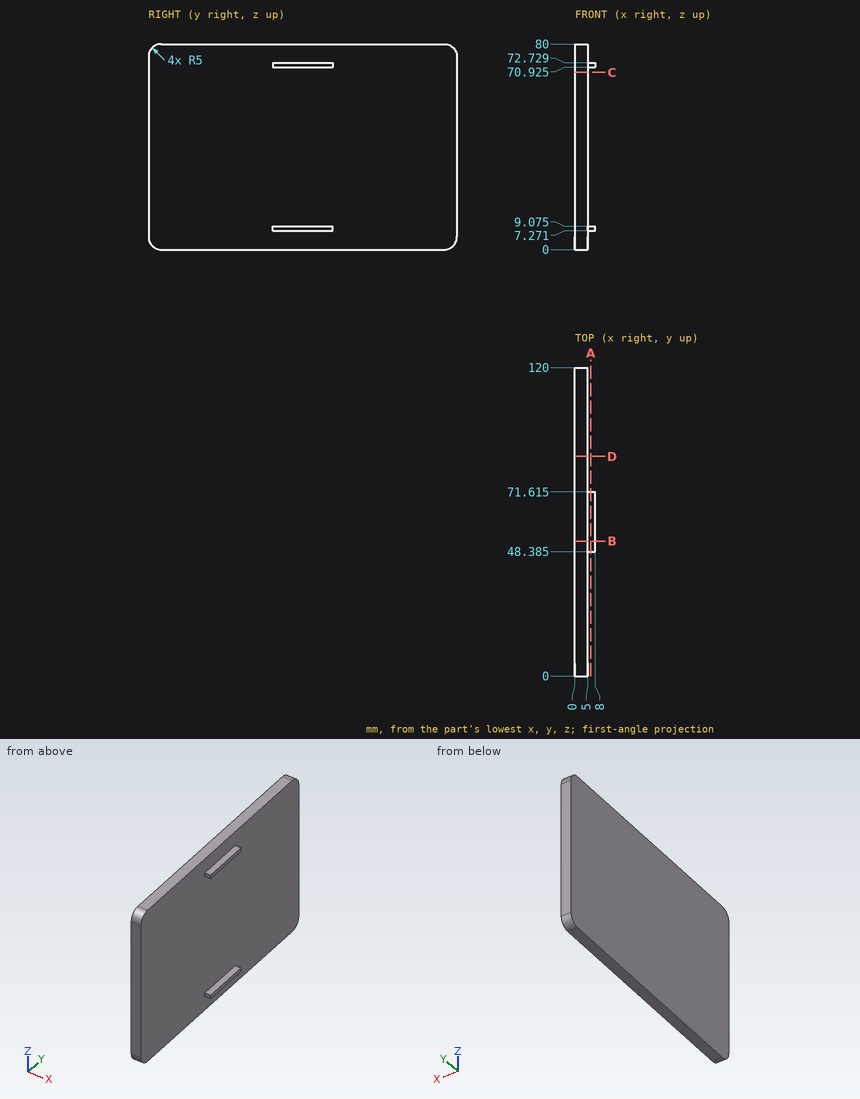
Job drawing, mm, ordinate dimensions from the low corner. One solid piece. Round coordinates to 2 decimals unless told otherwise and drop trailing zeros. Loops run counter-clockwise (first coordinate to the right, second up) from the corner with the lowest first, then second, coordinate; pieces in that order, holes last. Notation, with made-up numbers: (15.25, 2.5) -> (34.25, 2.5) arc R27 ccw to (34.25, 27.5) -> close; hole circle Ø2 at (73.25, 6). An arc over 180 degrees is marked (long way). Use a Markdown table: item, result.
1) Cut at A-A, the plane x = 6.25. List the corners of the cut face in (y, z) (1 decimal).
The answers:
| item | result |
|---|---|
| outline | (48.4, 7.3) -> (71.6, 7.3) -> (71.6, 9.1) -> (48.4, 9.1) -> close; (48.4, 70.9) -> (71.6, 70.9) -> (71.6, 72.7) -> (48.4, 72.7) -> close |
2) Cut at D-D, the plane y = 85.5. List the corners of the cut face in (x, z).
The answers:
| item | result |
|---|---|
| outline | (0, 0) -> (5, 0) -> (5, 80) -> (0, 80) -> close |
3) Cut at B-B, the plane y = 52.5. List the corners of the cut face in (x, z) (1 decimal).
The answers:
| item | result |
|---|---|
| outline | (0, 0) -> (5, 0) -> (5, 7.3) -> (8, 7.3) -> (8, 9.1) -> (5, 9.1) -> (5, 70.9) -> (8, 70.9) -> (8, 72.7) -> (5, 72.7) -> (5, 80) -> (0, 80) -> close |
4) Probe line 1 (X direction, y = 46, z = 32). List the from-to ranges inside material, lowest first. Write a range as [from, to].
The answers:
| item | result |
|---|---|
| line 1 | x = [0, 5] |
5) Drop flat-ended pins along their axis: pin 1 Ø0.5 at (x, z) = (6, 72) entering from -Y (1 decimal); pin 2 Ø0.5 at (x, z) = (7, 71.5) entering from +Y (1 decimal); pin 3 Ø1.5 at (x, y) = (6, 58) entering from -Z. Give the stop position or say it passes through.
The answers:
| item | result |
|---|---|
| pin 1 | stops at y = 48.4 |
| pin 2 | stops at y = 71.6 |
| pin 3 | stops at z = 7.27 |
6) Cut at C-C, the plane z = 69. List the corners of the cut face in (x, y).
The answers:
| item | result |
|---|---|
| outline | (0, 0) -> (5, 0) -> (5, 120) -> (0, 120) -> close |
